Design review of the part built by this model. Coordinates are the model's own, in mm. Face numbers are marked on the shaded views. A direction names the side the tool comes from. Give positions to 0.01 mm unless a question says otherwise; leave off trailing zeros. Write each loop counter-clockwise with the first axis right and the second up, starting at its lowest first coordinate (ties: lowest second). Pieces come first, ordered by that corner, then holes. Notation, with made-up numbers: (-4, -1.75) - (22, -1.75) arc R18 cw to (22, 18.25) - close; hole circle Ø7 at (60.25, 19.5). An arc over 180 degrees is marked (long way). Write each question's results on one line, items separated by ' | '. Start each with the question number.
from build123d import *

# Parameters (mm, degrees)
SKICA1_W                 = 11
SKICA1_H                 = 7.4
P_IDAT_VYSUNUT_M1_DEPTH  = 21
ODEBRAT_VYSUNUT_M1_DEPTH = 21
P_IDAT_VYSUNUT_M2_DEPTH  = 6


with BuildPart() as part:
    # Skica1 → Přidat vysunutím1 (new body)
    with BuildSketch(Plane.XY):
        Rectangle(SKICA1_W, SKICA1_H)
    extrude(amount=P_IDAT_VYSUNUT_M1_DEPTH)

    # Skica2 → Odebrat vysunutím1 (cut)
    with BuildSketch(Plane(origin=(0, 3.7, 0), x_dir=(1, 0, 0), z_dir=(0, 1, 0))):
        Polygon((-5.5, -11), (-3.75, -21), (3.75, -21), (5.5, -11), (8.02176331, -11), (9.220966656, -26.189909052), (-8.647163202, -26.189909052), align=None)
    extrude(amount=-ODEBRAT_VYSUNUT_M1_DEPTH, mode=Mode.SUBTRACT)

    # Skica3 → Přidat vysunutím2 (add)
    with BuildSketch(Plane(origin=(0, 0, 0), x_dir=(-1, 0, 0), z_dir=(0, 0, -1))):
        Polygon((-3.4, 0.1), (-2.6, 0.9), (2.6, 0.9), (3.4, 0.1), (3.4, -0.9), (-3.4, -0.9), align=None)
    extrude(amount=P_IDAT_VYSUNUT_M2_DEPTH)


solid = part.part
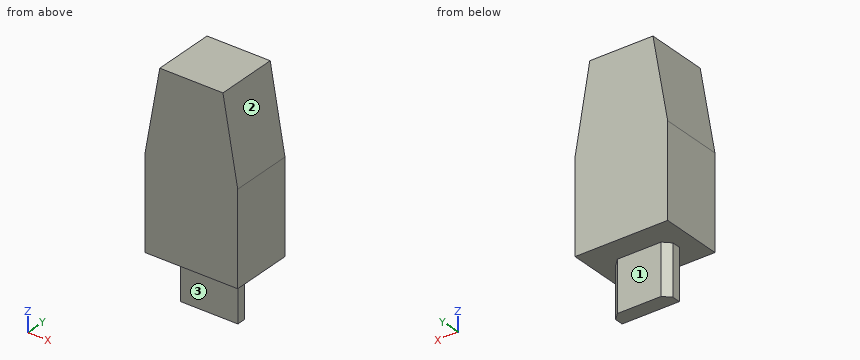
Q1. Add section D-D on y = 2.75. State the section outline as (x, z) points.
Q2. Insertion check: P1, Ø1.5, axis at x = 3, y = -2.5, coming from the -Z side; P2, Ø1.6, axis at x = 0, z = -2.5, coming from the +Y side; P3, Ø0.5, axis at y = -0.5, z = -2, coming from the +X side. Each pin has a flat end and moves straight along its axis. Give the tip position at first contact, or say it passes through.
Q3. Add section A-A on y = -0.5. State the section outline as (x, z) points.
Q4. For line 1 along Z through (x, y) = (-0.25, 3.5); line 2 along X through (y, z) = (0.75, 15); line 3 along X through (y, z) = (3.5, 14.25), list the stretches that pass through material, from the lowest coordinate up. Write a range as [from, to].
Q5. Add section C-C on z = -3.5. State the section outline as (x, y) points, plus the area to 3 significant figures.
Q6. Add section B-B on x = -1. State the section outline as (y, z) points, plus the area to 3 significant figures.
Q7. Machinability: for the marked faces 1, 2 and 3, which of the approach directions +Z, -Z, +X, -X, +Y, -Y give a long, thin tool a straight path to every point of the face, cutting with its end or side? Answer none if there is none.
Result:
1) outline: (-5.5, 0) - (5.5, 0) - (5.5, 11) - (3.75, 21) - (-3.75, 21) - (-5.5, 11) - close
2) P1: stops at z = 0 | P2: stops at y = 0.9 | P3: stops at x = 3.4
3) outline: (-5.5, 0) - (-3.4, 0) - (-3.4, -6) - (3.4, -6) - (3.4, 0) - (5.5, 0) - (5.5, 11) - (3.75, 21) - (-3.75, 21) - (-5.5, 11) - close
4) line 1: z = [0, 21] | line 2: x = [-4.8, 4.8] | line 3: x = [-4.93, 4.93]
5) outline: (-3.4, -0.9) - (3.4, -0.9) - (3.4, 0.1) - (2.6, 0.9) - (-2.6, 0.9) - (-3.4, 0.1) - close | area: 11.6 mm²
6) outline: (-3.7, 0) - (-0.9, 0) - (-0.9, -6) - (0.9, -6) - (0.9, 0) - (3.7, 0) - (3.7, 21) - (-3.7, 21) - close | area: 166 mm²
7) face 1: -Z, +X, -X, +Y | face 2: +Z, +X, +Y, -Y | face 3: -Z, +X, -X, -Y
